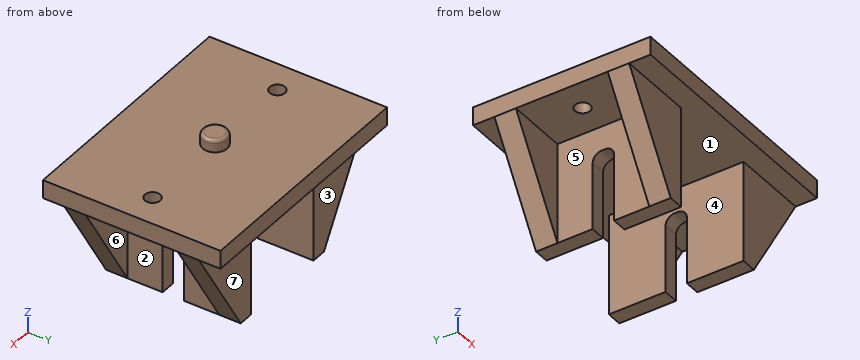
```python
from build123d import *

# Parameters (mm, degrees)
SKETCH_2_W               = 80
SKETCH_2_H               = 58
SKETCH_2_R               = 2.5
EXTRUDE_1_DEPTH          = 6
SKETCH_3_W               = 5
SKETCH_3_H               = 44
EXTRUDE_2_DEPTH          = 33
CUT_EXTRUDE_1_DEPTH      = 75.36396977
CUT_EXTRUDE_1_DEPTH_BACK = 75.36396977
SKETCH_12_R              = 4
EXTRUDE_3_DEPTH          = 4
RIB_10_REACH             = 70.007
SKETCH_13_WALL_W         = 176.60226785
SKETCH_13_WALL_H         = 7
RIB_12_REACH             = 70.007
SKETCH_16_WALL_W         = 176.60226785
SKETCH_16_WALL_H         = 7
FILLET_2_R               = 1


with BuildPart() as part:
    # 스케치2 → 보스-돌출1 (new body)
    with BuildSketch(Plane.XY):
        Rectangle(SKETCH_2_W, SKETCH_2_H)
        with Locations((-30, 0)):
            Circle(SKETCH_2_R, mode=Mode.SUBTRACT)
        with Locations((30, 0)):
            Circle(SKETCH_2_R, mode=Mode.SUBTRACT)
    extrude(amount=EXTRUDE_1_DEPTH)

    # 스케치3 → 보스-돌출2 (add)
    with BuildSketch(Plane(origin=(0, 0, 0), x_dir=(-1, 0, 0), z_dir=(0, 0, -1))):
        with Locations((-17.5, 0)):
            Rectangle(SKETCH_3_W, SKETCH_3_H)
        with Locations((17.5, 0)):
            Rectangle(SKETCH_3_W, SKETCH_3_H)
    extrude(amount=EXTRUDE_2_DEPTH)

    # 스케치11 → 컷-돌출1 (cut, two sides: drawn at the far end of the back side and taken through both)
    with BuildSketch(Plane(origin=(20, 0, 0), x_dir=(0, 0, -1), z_dir=(1, 0, 0)).offset(-CUT_EXTRUDE_1_DEPTH_BACK)):
        with BuildLine():
            Line((33, -3.5), (11, -3.5))
            ThreePointArc((11, -3.5), (8.878679656, -2.621320344), (8, -0.5))
            Line((8, -0.5), (8, 0.5))
            ThreePointArc((8, 0.5), (8.878679656, 2.621320344), (11, 3.5))
            Line((11, 3.5), (33, 3.5))
            Line((33, 3.5), (33, -3.5))
        make_face()
    extrude(amount=CUT_EXTRUDE_1_DEPTH + CUT_EXTRUDE_1_DEPTH_BACK, mode=Mode.SUBTRACT)

    # 스케치12 → 보스-돌출3 (add)
    with BuildSketch(Plane.XY.offset(6)):
        with Locations(Location((0, 0, 0), (0, 0, 180))):
            Circle(SKETCH_12_R)
    extrude(amount=EXTRUDE_3_DEPTH)

    # 스케치13 wall → 보강대10 (add, up to next)
    with BuildSketch(Plane(origin=(-30, 15, -16.5), x_dir=(-0.518301716093, 0, 0.855197831554), z_dir=(0.855197831554, 0, 0.518301716093)), mode=Mode.PRIVATE) as rib_10_sk1:
        with Locations((0, -3.5)):
            Rectangle(SKETCH_13_WALL_W, SKETCH_13_WALL_H)
    rib_10_tool1 = extrude(rib_10_sk1.sketch, amount=RIB_10_REACH, mode=Mode.PRIVATE) - part.part
    rib_10 = rib_10_tool1.solids().sort_by_distance((-30, 15, -16.5))[0]
    add(rib_10)

    # 스케치16 wall → 보강대12 (add, up to next)
    with BuildSketch(Plane(origin=(-30, -15, -16.5), x_dir=(-0.518301716093, 0, 0.855197831554), z_dir=(0.855197831554, 0, 0.518301716093)), mode=Mode.PRIVATE) as rib_12_sk1:
        with Locations((0, 3.5)):
            Rectangle(SKETCH_16_WALL_W, SKETCH_16_WALL_H)
    rib_12_tool1 = extrude(rib_12_sk1.sketch, amount=RIB_12_REACH, mode=Mode.PRIVATE) - part.part
    rib_12 = rib_12_tool1.solids().sort_by_distance((-30, -15, -16.5))[0]
    add(rib_12)

    # 대칭 복사1: 보강대10 across plane
    add(rib_10.mirror(Plane(origin=(0, 0, 0), x_dir=(0, 0, 1), z_dir=(1, 0, 0))))

    # 대칭 복사2: 보강대12 across plane
    add(rib_12.mirror(Plane(origin=(0, 0, 0), x_dir=(0, 0, 1), z_dir=(1, 0, 0))))

    # 필렛2
    fillet_2_edges = [part.edges().sort_by_distance(p)[0] for p in [
        (4, 0, 10),
    ]]
    fillet(fillet_2_edges, radius=FILLET_2_R)


solid = part.part
```
Model file for the job. Use its own axes, mm. Face numbers are marked on the shaded views. A direction names the side the tool comes from. Coordinates: 2 decimals unless noted, no trailing zeros. Order: outer loops, then holes, each group sorted by start corner. A loop starts at its lowest first (then second) coordinate and runs counter-clockwise, first axis right, second up. Notation, with made-up numbers: (81.5, -10) -> (131.5, -10) arc R18 ccw to (131.5, -5) -> close; hole circle Ø1 at (44, 77.25). An arc over 180 degrees is marked (long way). Answer as a JSON object with one key per item and string values. Group by question number.
1) Cut at D-D, the plane x = 0. Write the cut outline in (y, z).
2) Cut at C-C, the plane y = -11.5. Write the cut outline in (x, z), then the cut area to 3 significant figures.
3) Cut at B-B, the plane z = -16. Write the cut outline in (x, y).
4) Drill centre lines: L1, parallel to Y at x = 30, z = 2.4; L2, parallel to X at y = 7, z = -29.5; L3, parallel to Y at x = 29, z = -13. Where is each one in solid material? Low to high.
5) Which spindle directions (+Z, -Z, +X, -X, +Y, -Y) get a long thin tool onto all of the face, cutting with end or side? Do the marked faces 5, 6 and 7. Say none if no direction does.
6) Cut at A-A, the plane x = 30. Write the cut outline in (y, z), then the cut area to 3 significant figures.
7) Pull direction X, two halves, no side cores. Call the marked faces 1, 2, 3 and 4: +X half, -X half, draft (parallel to the pull), parting line (faces both ways), or undercut.
8) Flat gauge pins, fed straight in: pin 1 (0.8 mm diameter, centred on x = 18.5, y = 0, fed in from -Z); pin 2 (4 mm diameter, centred on y = 11.5, z = -3.5, fed in from -X); pin 3 (5 mm diameter, centred on x = 17.5, z = -10.5, fed in from +Y). Where does each tip first touch, or does it go through?
Check values:
{
 "1": {"outline": "(-29, 0) -> (29, 0) -> (29, 6) -> (4, 6) -> (4, 9) arc R1 ccw to (3, 10) -> (-3, 10) arc R1 ccw to (-4, 9) -> (-4, 6) -> (-29, 6) -> close"},
 "2": {"outline": "(-40, 0) -> (-20, 0) -> (-20, -33) -> (-15, -33) -> (-15, 0) -> (15, 0) -> (15, -33) -> (20, -33) -> (20, 0) -> (40, 0) -> (40, 6) -> (-40, 6) -> close", "area": "810 mm²"},
 "3": {"outline": "(-30.3, -22) -> (-15, -22) -> (-15, -3.5) -> (-20, -3.5) -> (-20, -15) -> (-30.3, -15) -> close; (-30.3, 15) -> (-20, 15) -> (-20, 3.5) -> (-15, 3.5) -> (-15, 22) -> (-30.3, 22) -> close; (15, -22) -> (30.3, -22) -> (30.3, -15) -> (20, -15) -> (20, -3.5) -> (15, -3.5) -> close; (15, 3.5) -> (20, 3.5) -> (20, 15) -> (30.3, 15) -> (30.3, 22) -> (15, 22) -> close"},
 "4": {"L1": "y = -29 to -2.5, 2.5 to 29", "L2": "x = -20 to -15, 15 to 20", "L3": "y = -22 to -15, 15 to 22"},
 "5": {"face 5": "-Z, -X", "face 6": "-Z, +X", "face 7": "-Z, +X, -X, +Y"},
 "6": {"outline": "(-29, 0) -> (-22, 0) -> (-22, -16.5) -> (-15, -16.5) -> (-15, 0) -> (-2.5, 0) -> (-2.5, 6) -> (-29, 6) -> close; (2.5, 0) -> (15, 0) -> (15, -16.5) -> (22, -16.5) -> (22, 0) -> (29, 0) -> (29, 6) -> (2.5, 6) -> close", "area": "549 mm²"},
 "7": {"face 1": "undercut", "face 2": "+X half", "face 3": "draft", "face 4": "undercut"},
 "8": {"pin 1": "stops at z = -8", "pin 2": "stops at x = -20", "pin 3": "stops at y = 22"}
}
